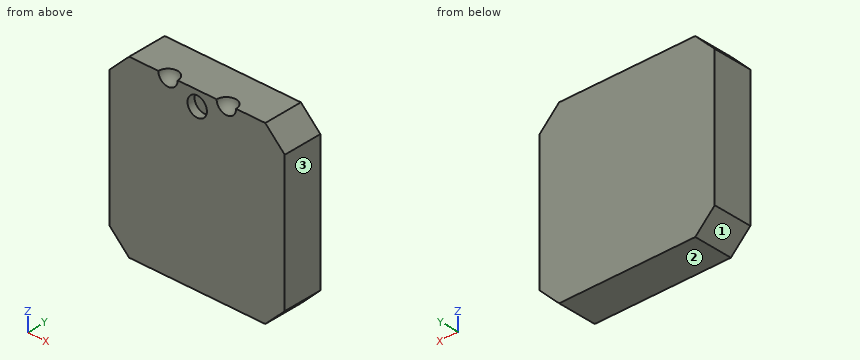
from build123d import *

# Parameters (mm, degrees)
SKETCH1_W           = 114.3
SKETCH1_H           = 114.3
BOSS_EXTRUDE1_DEPTH = 25.4
CHAMFER1_SIZE       = 12.7
SKETCH2_R           = 6.35
CUT_EXTRUDE1_DEPTH  = 5.08


with BuildPart() as part:
    # Sketch1 → Boss-Extrude1 (new body)
    with BuildSketch(Plane(origin=(0, 0, 0), x_dir=(1, 0, 0), z_dir=(0, 1, 0))):
        Rectangle(SKETCH1_W, SKETCH1_H)
    extrude(amount=BOSS_EXTRUDE1_DEPTH)

    # Chamfer1
    chamfer1_edges = [part.edges().sort_by_distance(p)[0] for p in [
        (57.15, 12.7, 57.15),
        (-57.15, 12.7, 57.15),
        (-57.15, 12.7, -57.15),
        (57.15, 12.7, -57.15),
    ]]
    chamfer(chamfer1_edges, length=CHAMFER1_SIZE)

    # Sketch2 → Cut-Extrude1 (cut)
    with BuildSketch(Plane(origin=(0, 0, 0), x_dir=(-1, 0, 0), z_dir=(0, -1, 0))):
        with Locations(Location((0, -47.625, 0), (0, 0, 90))):
            Circle(SKETCH2_R)
    extrude(amount=-CUT_EXTRUDE1_DEPTH, mode=Mode.SUBTRACT)

    # Sketch3 → Cut-Revolve4 (revolve, cut)
    with BuildSketch(Plane.XY.offset(57.15)):
        with BuildLine():
            Line((-25.4, 0), (-12.7, 0))
            ThreePointArc((-12.7, 0), (-19.05, 6.35), (-25.4, 0))
        make_face()
        with BuildLine():
            Line((25.4, 0), (12.7, 0))
            ThreePointArc((12.7, 0), (19.05, 6.35), (25.4, 0))
        make_face()
    revolve(axis=Axis((-57.15, 0, 57.15), (1, 0, 0)), mode=Mode.SUBTRACT)


solid = part.part
Build history of the part. All positions in model axes, mm. Face numbers are marked on the shaded views. Give positions to 0.01 mm unless a question says otherwise; leave off trailing zeros. Order: outer loops, then holes, each group sorted by start corner. A loop starts at its lowest first (then second) coordinate and runs counter-clockwise, first axis right, second up. Notation, with made-up numbers: M 38,61.5 L 96,61.5 A28 cw 96,99.5 Z; hole C 89.25,70.25 d5. An arc over 180 degrees is marked long. Put each result on its own line as item: value.
Item 1: Probe line 1 (X direction, y = 4.25, z = 46); line 2 (Y direction, x = 2, z = 50.5); line 3 (X direction, y = 10.5, z = 46). List the from-to ranges inside material, lowest first. Write a range as [from, to].
From the geometry:
line 1: x = [-55.6, -6.14], [6.14, 55.6]
line 2: y = [5.08, 25.4]
line 3: x = [-55.6, 55.6]
Item 2: Two-plate mould, pull along X, no slides. Class the marked faces 1, 2 and 3: +X half, -X half, draft (parallel to the pull), parting line (faces both ways), or undercut.
From the geometry:
face 1: -X half
face 2: draft
face 3: +X half
Item 3: Flat gauge pins, fed straight in: pin 1 Ø6.5 at (x, z) = (2.5, 49) entering from -Y; pin 2 Ø1.5 at (x, y) = (-45.5, 6) entering from -Z. Where does each tip first touch, or does it go through?
From the geometry:
pin 1: stops at y = 5.08
pin 2: stops at z = -56.85
Item 4: Slice it at B-B, the plane y = 12.5. Write the cut outline in (x, z), plus the area to 3 significant figures.
From the geometry:
outline: M -57.15,-44.45 L -44.45,-57.15 L 44.45,-57.15 L 57.15,-44.45 L 57.15,44.45 L 44.45,57.15 L -44.45,57.15 L -57.15,44.45 Z
area: 12,700 mm2
Item 5: Slice it at A-A, the plane x = 0. Write the cut outline in (y, z) (3 decimals).
From the geometry:
outline: M 0,-57.15 L 25.4,-57.15 L 25.4,57.15 L 0,57.15 L 0,53.975 L 5.08,53.975 L 5.08,41.275 L 0,41.275 Z
